Work out the finished part from the listing and answer in its coordinate system (mm). Give positions to 0.01 mm unless a question says otherwise; leave off trailing zeros. Loops run counter-clockwise (first coordinate to the right, second up) from the corner with the lowest first, then second, coordinate; pieces in that order, holes last. Notation, with made-up numbers: M 59.5,78 L 76.5,78 A26 cw 76.5,93 Z; hole C -3.75,29 d5. An arc over 180 degrees is marked long. Use a Markdown table: item, result.
```python
from build123d import *

# Parameters (mm, degrees)
F0_R     = 2.5
F1_DEPTH = 1.6


with BuildPart() as f1:
    # F0 (on Top) → F1 (new body)
    with BuildSketch(Plane.XY):
        with BuildLine():
            ThreePointArc((16.5, 73.5), (15.035534, 69.964466), (11.5, 68.5))
            Line((11.5, 68.5), (3.5, 68.5))
            Line((3.5, 68.5), (3.5, 16.5))
            Line((3.5, 16.5), (11.5, 16.5))
            ThreePointArc((11.5, 16.5), (15.035534, 15.035534), (16.5, 11.5))
            Line((16.5, 11.5), (16.5, 7.75))
            Line((16.5, 7.75), (21.75, 7.75))
            Line((21.75, 7.75), (21.75, 4))
            Line((21.75, 4), (21.75, 2.5))
            Line((21.75, 2.5), (103.25, 2.5))
            Line((103.25, 2.5), (103.25, 4))
            Line((103.25, 4), (103.25, 7.75))
            Line((103.25, 7.75), (108.5, 7.75))
            Line((108.5, 7.75), (108.5, 11.5))
            ThreePointArc((108.5, 11.5), (109.964466, 15.035534), (113.5, 16.5))
            Line((113.5, 16.5), (121.5, 16.5))
            Line((121.5, 16.5), (121.5, 68.5))
            Line((121.5, 68.5), (113.5, 68.5))
            ThreePointArc((113.5, 68.5), (109.964466, 69.964466), (108.5, 73.5))
            Line((108.5, 73.5), (108.5, 77.25))
            Line((108.5, 77.25), (103.25, 77.25))
            Line((103.25, 77.25), (103.25, 81))
            Line((103.25, 81), (103.25, 82.5))
            Line((103.25, 82.5), (21.75, 82.5))
            Line((21.75, 82.5), (21.75, 81))
            Line((21.75, 81), (21.75, 77.25))
            Line((21.75, 77.25), (16.5, 77.25))
            Line((16.5, 77.25), (16.5, 73.5))
        make_face()
        with Locations((19, 19)):
            Circle(F0_R, mode=Mode.SUBTRACT)
        with Locations((106, 19)):
            Circle(F0_R, mode=Mode.SUBTRACT)
        with Locations((19, 66)):
            Circle(F0_R, mode=Mode.SUBTRACT)
        with Locations((106, 66)):
            Circle(F0_R, mode=Mode.SUBTRACT)
    extrude(amount=F1_DEPTH)


solid = f1.part
```
(1) A cutting plane is placed at C-C (x = 19). Write down the section's boundary in (y, z).
Entries:
| item | result |
|---|---|
| outline | M 7.75,0 L 16.5,0 L 16.5,1.6 L 7.75,1.6 Z; M 21.5,0 L 63.5,0 L 63.5,1.6 L 21.5,1.6 Z; M 68.5,0 L 77.25,0 L 77.25,1.6 L 68.5,1.6 Z |
(2) A cutting plane is placed at B-B (z = 0.4). Write down the section's boundary in (x, y).
Entries:
| item | result |
|---|---|
| outline | M 3.5,16.5 L 11.5,16.5 A5 cw 16.5,11.5 L 16.5,7.75 L 21.75,7.75 L 21.75,2.5 L 103.25,2.5 L 103.25,7.75 L 108.5,7.75 L 108.5,11.5 A5 cw 113.5,16.5 L 121.5,16.5 L 121.5,68.5 L 113.5,68.5 A5 cw 108.5,73.5 L 108.5,77.25 L 103.25,77.25 L 103.25,82.5 L 21.75,82.5 L 21.75,77.25 L 16.5,77.25 L 16.5,73.5 A5 cw 11.5,68.5 L 3.5,68.5 Z; hole C 19,19 d5; hole C 19,66 d5; hole C 106,19 d5; hole C 106,66 d5 |
(3) A cutting plane is placed at D-D (y = 76). Write down the section's boundary in (x, z), and give its area (3 significant figures).
Entries:
| item | result |
|---|---|
| outline | M 16.5,0 L 108.5,0 L 108.5,1.6 L 16.5,1.6 Z |
| area | 147 mm² |
(4) Given P1, Ø0.5, axis at x = 104.5, z = 0.5, coming from the +Y side; P2, Ø0.8, axis at y = 80, z = 1, coming from the +X side; P3, Ø0.8, axis at y = 9, z = 1, coming from the -X side, each flat-ended and moving along its own axis, determine where each tip first touches the part or whether it passes through.
Entries:
| item | result |
|---|---|
| P1 | stops at y = 77.25 |
| P2 | stops at x = 103.25 |
| P3 | stops at x = 16.5 |
(5) The mould has two halves that part along Y. Classify faces 1 (the cylindrical face through (15, 15.07, 0.79)), 2 (the cylindrical face through (110, 69.93, 0.79)), 3 (the flat face through (62, 43, 0)), 4 (the cylindrical face through (17.16, 20.69, 0.79)): released by +Y, released by -Y, zero draft, split by the parting line, or undercut.
Entries:
| item | result |
|---|---|
| face 1 | released by -Y |
| face 2 | released by +Y |
| face 3 | zero draft |
| face 4 | undercut |
(6) Consider probe 1 along Y at (x, z) = (19, 1.2); probe 2 along X at (y, z) = (14, 0.2); probe 3 along Y at (x, z) = (110, 0.8). Determine where each line is inside the solid, lowest interval first. Write a range as [from, to].
Entries:
| item | result |
|---|---|
| probe 1 | y = [7.75, 16.5], [21.5, 63.5], [68.5, 77.25] |
| probe 2 | x = [15.83, 109.17] |
| probe 3 | y = [15.07, 69.93] |
(7) A cutting plane is placed at A-A (y = 19). Write down the section's boundary in (x, z), and give its area (3 significant figures).
Entries:
| item | result |
|---|---|
| outline | M 3.5,0 L 16.5,0 L 16.5,1.6 L 3.5,1.6 Z; M 21.5,0 L 103.5,0 L 103.5,1.6 L 21.5,1.6 Z; M 108.5,0 L 121.5,0 L 121.5,1.6 L 108.5,1.6 Z |
| area | 173 mm² |
